from build123d import *

# Parameters (mm, degrees)
F0_R     = 0.9816666667
F1_DEPTH = 11
F2_R     = 0.7843333333
F3_DEPTH = 7
F4_SIZE  = 0.1
F5_SIZE2 = 0.1339745962
F5_SIZE  = 0.5
F6_W     = 0.7
F6_H     = 0.6
F7_DEPTH = 1
F8_SCALE = 3


with BuildPart() as f1:
    # F0 (on Top) → F1 (new body)
    with BuildSketch(Plane.XY):
        Circle(F0_R)
    extrude(amount=F1_DEPTH)

    # F2 (on face) → F3 (join)
    with BuildSketch(Plane.XY.offset(11)):
        Circle(F2_R)
    extrude(amount=F3_DEPTH)

    # F4
    f4_edges = [f1.edges().sort_by_distance(p)[0] for p in [
        (-0.981667, 0, 0),
    ]]
    chamfer(f4_edges, length=F4_SIZE)

    # F5
    f5_edges = [f1.edges().sort_by_distance(p)[0] for p in [
        (-0.784333, 0, 18),
    ]]
    f5_side = f1.faces().sort_by_distance((-0.784333, 0, 14.5))[0]
    chamfer(f5_edges, length=F5_SIZE, length2=F5_SIZE2, reference=f5_side)

    # F6 (on Front) → F7 (cut, symmetric)
    with BuildSketch(Plane.XZ):
        with Locations((-0.65, 0.3)):
            Rectangle(F6_W, F6_H)
    extrude(amount=F7_DEPTH, both=True, mode=Mode.SUBTRACT)


with BuildPart() as f1_1:
    # F8: moved
    add(f1.part.scale(F8_SCALE))


solid = f1_1.part
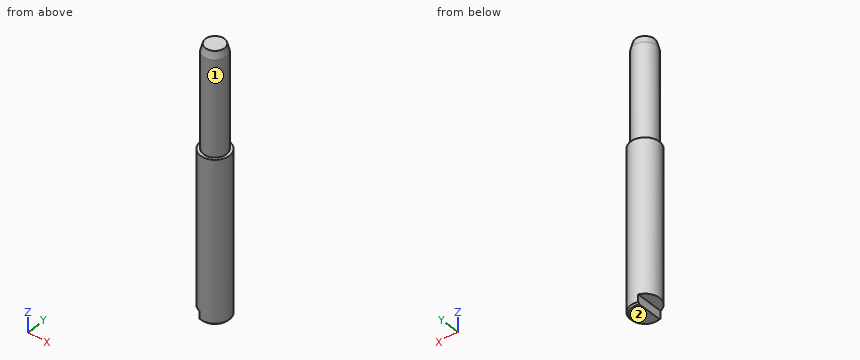
The listing builds one solid part. Answer for the finished solid, in the listing's coordinates (mm). Face numbers are marked on the shaded views. Give positions to 0.01 mm unless a question says otherwise; leave off trailing zeros. Write each loop counter-clockwise with the first axis right and the second up, starting at its lowest first coordinate (ties: lowest second). Pieces come first, ordered by that corner, then holes. Notation, with made-up numbers: (18, 21.25) -> (75, 21.25) arc R27 ccw to (75, 38.25) -> close; hole circle Ø8 at (41.25, 29.5). An arc over 180 degrees is marked (long way). Use a Markdown table: item, result.
(1) Section C-C, the plane z = 27.5 is taken. Determine the outline of the cut face in (x, y) (3 decimals), then the cut area to 3 significant figures.
Return value:
| item | result |
|---|---|
| outline | circle Ø5.89 at (0, 0) |
| area | 27.2 mm2 |
(2) Determine the mould class of the marked faces 1 and 2 for opening direction Y: released by +Y, released by -Y, zero draft, split by the parting line, or undercut.
Return value:
| item | result |
|---|---|
| face 1 | split by the parting line |
| face 2 | zero draft |
(3) Find the intervals of material crossed by probe 1 along Z at (x, y) = (1.95, -1.6); probe 2 along Z at (x, y) = (-1.3, 0.5); probe 3 along X at (y, z) = (0.05, 50), in increasing order. Write a range as from..to.
Return value:
| item | result |
|---|---|
| probe 1 | 0..33 |
| probe 2 | 1.8..54 |
| probe 3 | -2.35..2.35 |
(4) Section A-A, the plane x = 0 is taken. Determine the outline of the cut face in (y, z) (3 decimals), then the cut area to 3 significant figures.
Return value:
| item | result |
|---|---|
| outline | (-2.945, 0.3) -> (-2.645, 0) -> (2.645, 0) -> (2.945, 0.3) -> (2.945, 33) -> (2.353, 33) -> (2.353, 52.5) -> (1.951, 54) -> (-1.951, 54) -> (-2.353, 52.5) -> (-2.353, 33) -> (-2.945, 33) -> close |
| area | 293 mm2 |
(5) Flat-ended cylindrical pins translate along their axes: P1, Ø2, axis at y = -1, z = 1, coming from the -X side; P2, Ø1.5, axis at y = 0.5, z = 43.5, coming from the -X side; P3, Ø0.6, axis at x = -2.5, y = 0.5, coming from the -Z side. Find the tip coordinate at first contact, or state that the pin passes through.
Return value:
| item | result |
|---|---|
| P1 | x = -2.92 |
| P2 | x = -2.35 |
| P3 | z = 1.8 |
(6) Section D-D, the plane z = 49.5 is taken. Determine the outline of the cut face in (x, y), then the cut area to 3 significant figures.
Return value:
| item | result |
|---|---|
| outline | circle Ø4.71 at (0, 0) |
| area | 17.4 mm2 |
(7) Section B-B, the plane y = 0 is taken. Determine the outline of the cut face in (x, z) (3 decimals).
Return value:
| item | result |
|---|---|
| outline | (-2.945, 1.8) -> (-0.9, 1.8) -> (-0.9, 0) -> (2.645, 0) -> (2.945, 0.3) -> (2.945, 33) -> (2.353, 33) -> (2.353, 52.5) -> (1.951, 54) -> (-1.951, 54) -> (-2.353, 52.5) -> (-2.353, 33) -> (-2.945, 33) -> close |
